Read the model definition and answer for the solid it produces. Units are mm, in the model's axes. Coordinates: 2 decimals unless noted, no trailing zeros. Write each loop counter-clockwise with the first axis right and the second up, starting at its lowest first coordinate (ties: lowest second). Pieces come first, ordered by that corner, then holes.
Item 1: Straight lines are drawn through the part: probe 1 along X at (y, z) = (0.5, -60); probe 2 along X at (y, z) = (2.15, -90); probe 3 along Z at (x, y) = (11, 1.9). For each, find the intervals that lie inside material, in ascending order.
Item 2: Each of these flat-tipped pins is pushed along its axis until it touches: P1, Ø1.5, axis at x = -0.5, z = 8.5, coming from the -Y side; P2, Ø5, axis at x = 0, z = 57, coming from the +Y side. Where does it stop, or does it pass through?
Item 3: Section A-A (z = -90) is taken. Give the vertices of the cut face in (x, y), then the cut area to 3 significant figures.
from build123d import *

# Parameters (mm, degrees)
SKETCH1_W           = 40
SKETCH1_H           = 200
SKETCH1_R           = 2.6
SKETCH1_R_2         = 1.6
BOSS_EXTRUDE1_DEPTH = 3
CHAMFER1_SIZE       = 2


with BuildPart() as part:
    # Sketch1 → Boss-Extrude1 (new body)
    with BuildSketch(Plane(origin=(0, 0, 0), x_dir=(1, 0, 0), z_dir=(0, 1, 0))):
        Rectangle(SKETCH1_W, SKETCH1_H)
        with Locations((10, -90)):
            Circle(SKETCH1_R, mode=Mode.SUBTRACT)
        with Locations((10, 90)):
            Circle(SKETCH1_R, mode=Mode.SUBTRACT)
        with Locations((10, 60)):
            Circle(SKETCH1_R_2, mode=Mode.SUBTRACT)
        with Locations((-8, 60)):
            Circle(SKETCH1_R_2, mode=Mode.SUBTRACT)
        with Locations((0, -57)):
            Circle(SKETCH1_R_2, mode=Mode.SUBTRACT)
    extrude(amount=BOSS_EXTRUDE1_DEPTH)

    # Chamfer1
    chamfer1_edges = [part.edges().sort_by_distance(p)[0] for p in [
        (8.4, 3, -60),
        (-9.6, 3, -60),
        (-1.6, 3, 57),
    ]]
    chamfer(chamfer1_edges, length=CHAMFER1_SIZE)


solid = part.part
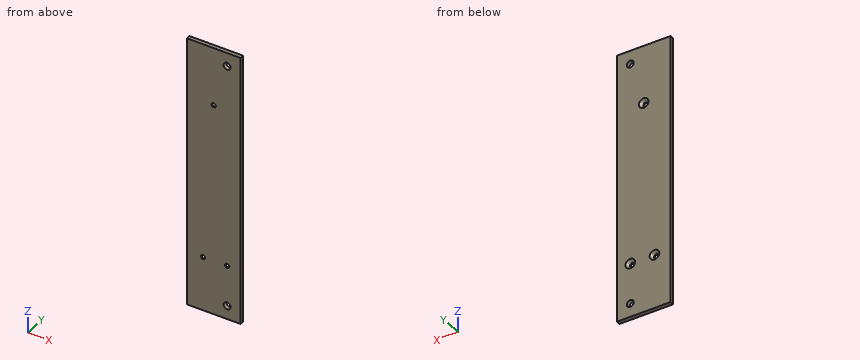
Established:
1. probe 1: x = -20 to -9.6, -6.4 to 8.4, 11.6 to 20
1. probe 2: x = -20 to 7.4, 12.6 to 20
1. probe 3: z = -100 to -92.4, -87.6 to -62.29, -57.71 to 87.6, 92.4 to 100
2. P1: stops at y = 0
2. P2: stops at y = 1.9
3. outline: (-20, 0) - (7.4, 0) - (7.4, 3) - (-20, 3) - close; (12.6, 0) - (20, 0) - (20, 3) - (12.6, 3) - close
3. area: 104 mm2
